Here's how the part is built. I have some questions about the finished solid (model axes, mm). Face numbers are marked on the shaded views. A direction names the side the tool comes from. Round coordinates to 2 decimals unless told otherwise and drop trailing zeros. Write each loop counter-clockwise with the first axis right and the second up, starting at its lowest first coordinate (ties: lowest second). Pieces come first, ordered by that corner, then holes. Notation, with made-up numbers: (3.25, 34) -> (37.25, 34) arc R20 ccw to (37.25, 46) -> close; hole circle Ø10 at (-10, -24.5). An arc over 180 degrees is marked (long way). Put each result on its own line as item: value. Start each with the question number.
1) Will these pins go through, and if not, where does the flat tip stop? P1, Ø1.4, axis at x = -13.84, z = -11.96, coming from the -Y side; P2, Ø1, axis at x = 12.5, y = 1.5, coming from the -Z side; P3, Ø1.5, axis at x = 12.5, y = 1.5, coming from the -Z side; P4, Ø1.6, axis at y = 1, z = -1.5, coming from the +X side.
2) I want a section at D-D, the plane y = 1.5. List the corners of the cut face in (x, z) for me, then the cut area to 3 significant figures.
3) I want a section at B-B, the plane z = -12.25. List the corners of the cut face in (x, y) for me (3 decimals), then the cut area to 3 significant figures.
4) I want a section at A-A, the plane x = -9. List the corners of the cut face in (y, z) for me (1 decimal).
5) I want a section at C-C, the plane z = -7.75. List the corners of the cut face in (x, y) for me (3 decimals), then the cut area to 3 significant figures.
6) If I drill on line 1 along X through (y, z) = (0.6, -11.25); line 2 along Z through (x, y) = (0.5, 1.8); line 3 along X through (y, z) = (0.65, -8), over which ranges is the centre line in solid material (lowest first)? Write a range as [from, to].
7) We'd pull the mould along X, two halves only. Please class the marked faces 4, 5 and 6: released by +X, released by -X, zero draft, split by the parting line, or undercut.
8) Which directions (+Z, -Z, +X, -X, +Y, -Y) give clear straight access to the entire face, cutting with the end or side of a thin tool? Please do the marked faces 1, 2 and 3.
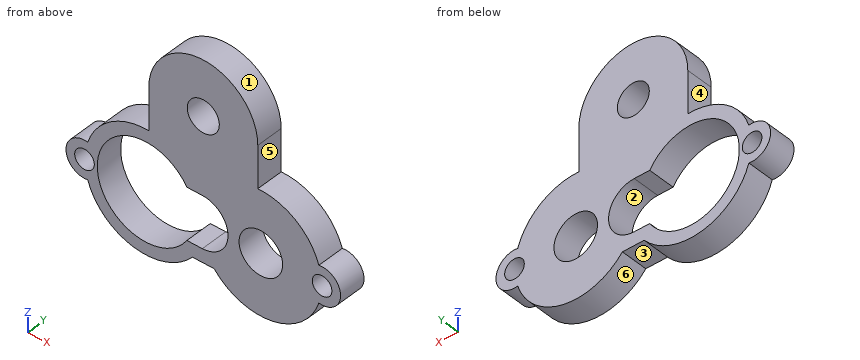
from build123d import *

# Parameters (mm, degrees)
SKETCH1_R           = 1.143
SKETCH1_R_2         = 1.8669
BOSS_EXTRUDE1_DEPTH = 3.175
SKETCH2_R           = 2.54
CUT_EXTRUDE1_DEPTH  = 26.080811969


with BuildPart() as part:
    # Sketch1 → Boss-Extrude1 (new body)
    with BuildSketch(Plane(origin=(0, 0, 0), x_dir=(1, 0, 0), z_dir=(0, 1, 0))):
        with BuildLine():
            ThreePointArc((13.466066475, 14.089241508), (16.002, 11.9634), (13.466066475, 9.837558492))
            ThreePointArc((13.466066475, 9.837558492), (10.753575803, 6.146552641), (6.35, 4.885739418))
            Line((6.35, 4.885739418), (6.35, 0))
            ThreePointArc((6.35, 0), (0, -6.35), (-6.35, 0))
            Line((-6.35, 0), (-6.35, 4.885739418))
            ThreePointArc((-6.35, 4.885739418), (-10.753575803, 6.146552641), (-13.466066475, 9.837558492))
            ThreePointArc((-13.466066475, 9.837558492), (-16.002, 11.9634), (-13.466066475, 14.089241508))
            ThreePointArc((-13.466066475, 14.089241508), (-8.085518963, 18.914398366), (-1.27, 16.51))
            Line((-1.27, 16.51), (1.27, 16.51))
            ThreePointArc((1.27, 16.51), (8.085518963, 18.914398366), (13.466066475, 14.089241508))
        make_face()
        with Locations(Location((13.843, 11.9634, 0), (0, 0, 270))):
            Circle(SKETCH1_R, mode=Mode.SUBTRACT)
        with Locations(Location((-13.843, 11.9634, 0), (0, 0, 270))):
            Circle(SKETCH1_R, mode=Mode.SUBTRACT)
        with Locations(Location((0, 0, 0), (0, 0, 270))):
            Circle(SKETCH1_R_2, mode=Mode.SUBTRACT)
    extrude(amount=BOSS_EXTRUDE1_DEPTH)

    # Sketch2 → Cut-Extrude1 (cut, through all)
    with BuildSketch(Plane(origin=(0, 3.175, 0), x_dir=(1, 0, 0), z_dir=(0, 1, 0))):
        with Locations(Location((6.705837378, 11.9634, 0), (0, 0, 270))):
            Circle(SKETCH2_R)
        with BuildLine():
            Line((-0.114537378, 8.9662), (-1.914569862, 8.9662))
            ThreePointArc((-1.914569862, 8.9662), (-12.357337378, 11.9634), (-1.914569862, 14.9606))
            Line((-1.914569862, 14.9606), (-0.114537378, 14.9606))
            ThreePointArc((-0.114537378, 14.9606), (2.882662622, 11.9634), (-0.114537378, 8.9662))
        make_face()
    extrude(amount=-CUT_EXTRUDE1_DEPTH, mode=Mode.SUBTRACT)


solid = part.part
Findings:
1. P1: passes through
1. P2: stops at z = -16.67
1. P3: stops at z = -16.94
1. P4: stops at x = 6.35
2. outline: (-13.47, -14.09) arc R7.09 ccw to (-1.27, -16.51) -> (1.27, -16.51) arc R7.09 ccw to (13.47, -14.09) arc R2.16 ccw (long way) to (13.47, -9.84) arc R7.09 ccw to (6.35, -4.89) -> (6.35, 0) arc R6.35 ccw to (-6.35, 0) -> (-6.35, -4.89) arc R7.09 ccw to (-13.47, -9.84) arc R2.16 ccw (long way) to start; hole circle Ø2.29 at (-13.84, -11.96); hole (-1.91, -14.96) -> (-0.11, -14.96) arc R3 ccw to (-0.11, -8.97) -> (-1.91, -8.97) arc R5.65 ccw (long way) to start; hole circle Ø3.73 at (0, 0); hole circle Ø5.08 at (6.71, -11.96); hole circle Ø2.29 at (13.84, -11.96)
2. area: 313 mm2
3. outline: (-15.983, 0) -> (-14.949, 0) -> (-14.949, 3.175) -> (-15.983, 3.175) -> close; (-12.737, 0) -> (-12.35, 0) -> (-12.35, 3.175) -> (-12.737, 3.175) -> close; (2.869, 0) -> (4.182, 0) -> (4.182, 3.175) -> (2.869, 3.175) -> close; (9.23, 0) -> (12.737, 0) -> (12.737, 3.175) -> (9.23, 3.175) -> close; (14.949, 0) -> (15.983, 0) -> (15.983, 3.175) -> (14.949, 3.175) -> close
3. area: 23.1 mm2
4. outline: (0, -18.7) -> (3.2, -18.7) -> (3.2, -17.1) -> (0, -17.1) -> close; (0, -6.8) -> (3.2, -6.8) -> (3.2, -5.3) -> (0, -5.3) -> close
5. outline: (-12.404, 0) -> (-10.472, 0) -> (-10.472, 3.175) -> (-12.404, 3.175) -> close; (-2.939, 0) -> (12.404, 0) -> (12.404, 3.175) -> (-2.939, 3.175) -> close
5. area: 54.8 mm2
6. line 1: x = [-15.88, -14.74], [-12.95, -12.31], [2.8, 4.27], [9.14, 12.95], [14.74, 15.88]
6. line 2: z = [-16.51, -14.9], [-9.03, -1.8], [1.8, 6.33]
6. line 3: x = [-12.58, -10.73], [-2.68, 12.58]
7. face 4: released by -X
7. face 5: released by +X
7. face 6: undercut
8. face 1: +Z, +Y, -Y
8. face 2: +Y, -Y
8. face 3: -Z, +Y, -Y
